Geometry: final body of the model. Coordinates: model frame, mm. Face numbers are marked on the shaded views. Round coordinates to 2 decimals unless told otherwise and drop trailing zeros. Loops run counter-clockwise (first coordinate to the right, second up) from the corner with the lowest first, then second, coordinate; pieces in that order, holes last. Notation, with made-up numbers: (23, 27.5) - (56, 27.5) arc R11 ccw to (56, 44.5) - close; hole circle Ø9 at (-20, 12). An arc over 180 degrees is marked (long way). Return JSON: item names as keys, results as strings. Group by question number.
1. Material intervals for probe 1 along X at (y, z) = (43.5, 21); probe 2 along Y at (x, z) = (20, 5); probe 3 along Y at (x, z) = (-20, 21), sorted ascending.
2. Section A-A on x = 20. Return loops of the section in (y, z), and give its area (3 significant figures).
3. Section D-D on x = -2. Return loops of the section in (y, z), and give its area (3 significant figures).
4. Section C-C on y = -2. Return loops of the section in (x, z).
5. Section B-B on y = -90. Count the separate pieces of the cut face and the enclosed holes in it, and give its area (3 significant figures).
6. Draft query along Z for the marked faces 1, 2 and 3. Return one class per face: +Z half, -Z half, draft (parallel to the pull), parting line (faces both ways), or undercut.
from build123d import *

# Parameters (mm, degrees)
F1_DEPTH       = 120
F3_D           = 8.5
F3_CBORE_D     = 14
F3_CBORE_DEPTH = 10


with BuildPart() as f1:
    # F0 (on Front) → F1 (new body, symmetric)
    with BuildSketch(Plane.XZ):
        Polygon((-55, 26), (-55, 0), (55, 0), (55, 26), (46, 26), (46, 18), (50, 18), (50, 10), (30, 10), (30, 18.192771), (34, 18.192771), (34, 26), (6, 26), (6, 18), (10, 18), (10, 10), (-10, 10), (-10, 18.192771), (-6, 18.192771), (-6, 26), (-34, 26), (-34, 18), (-30, 18), (-30, 10), (-50, 10), (-50, 18.192771), (-46, 18.192771), (-46, 26), align=None)
    extrude(amount=F1_DEPTH, both=True)

    # F3 (through all)
    with Locations(Plane.XY.offset(26)):
        with Locations((-20, -90), (20, -90), (-20, 90), (20, 90)):
            CounterBoreHole(F3_D / 2, F3_CBORE_D / 2, F3_CBORE_DEPTH)


with BuildPart() as f4_1:
    # F4: copy of F1
    add(f1.part)


solid = f1.part
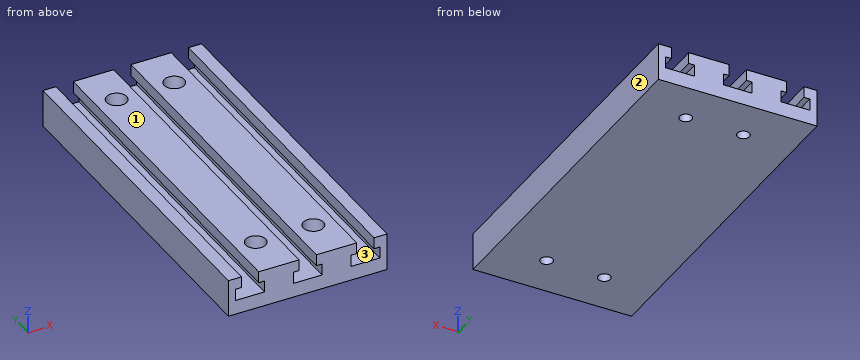
Taken from the geometry:
{
 "1": {"probe 1": "-55 to -46, -34 to -6, 6 to 34, 46 to 55", "probe 2": "-120 to -94.25, -85.75 to 85.75, 94.25 to 120", "probe 3": "-120 to -97, -83 to 83, 97 to 120"},
 "2": {"outline": "(-120, 0) - (-94.25, 0) - (-94.25, 16) - (-97, 16) - (-97, 26) - (-120, 26) - close; (-85.75, 0) - (85.75, 0) - (85.75, 16) - (83, 16) - (83, 26) - (-83, 26) - (-83, 16) - (-85.75, 16) - close; (94.25, 0) - (120, 0) - (120, 26) - (97, 26) - (97, 16) - (94.25, 16) - close", "area": "5,690 mm2"},
 "3": {"outline": "(-120, 0) - (120, 0) - (120, 10) - (-120, 10) - close", "area": "2,400 mm2"},
 "4": {"outline": "(-55, 0) - (55, 0) - (55, 26) - (46, 26) - (46, 18) - (50, 18) - (50, 10) - (30, 10) - (30, 18.19) - (34, 18.19) - (34, 26) - (6, 26) - (6, 18) - (10, 18) - (10, 10) - (-10, 10) - (-10, 18.19) - (-6, 18.19) - (-6, 26) - (-34, 26) - (-34, 18) - (-30, 18) - (-30, 10) - (-50, 10) - (-50, 18.19) - (-46, 18.19) - (-46, 26) - (-55, 26) - close"},
 "5": {"separate pieces": "3", "enclosed holes": "0", "area": "1,540 mm2"},
 "6": {"face 1": "+Z half", "face 2": "draft", "face 3": "undercut"}
}
